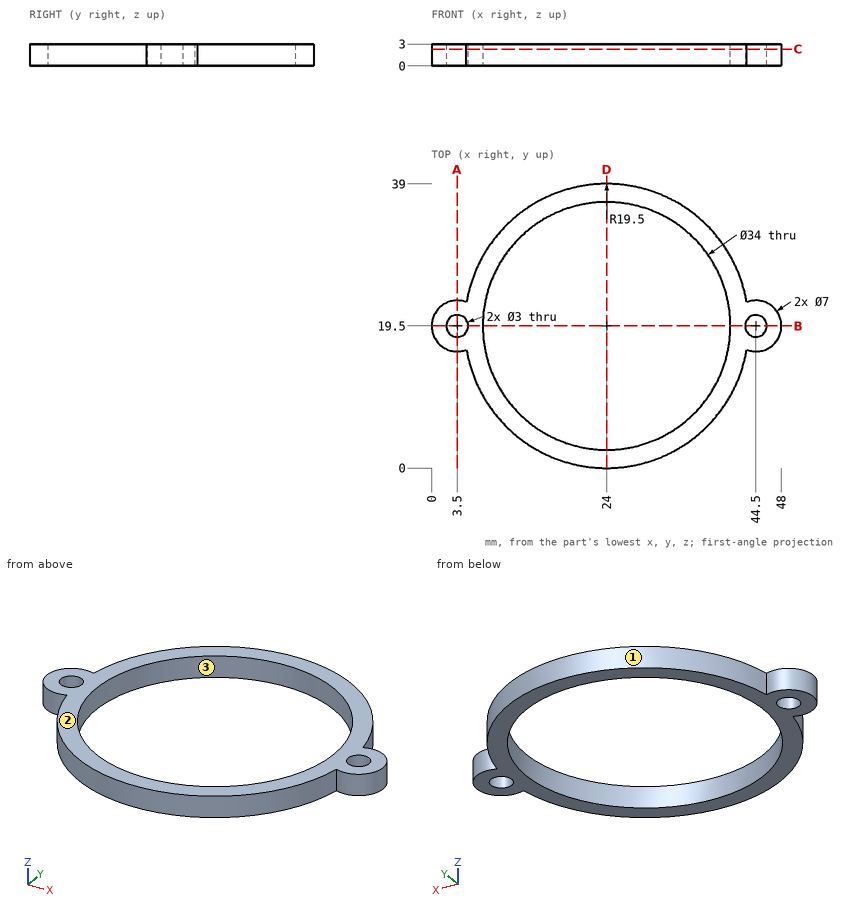
The figure shows three views and two pictorial views of one solid part (mm, origin at its lowest corner). Answer the questions. Coordinates: 2 decimals unless noted, no trailing zeros. Loops run counter-clockwise (first coordinate to the right, second up) from the corner with the lowest first, then second, coordinate; pieces in that order, holes last. Notation, with made-up numbers: (52.5, -16) -> (76.5, -16) arc R18 cw to (76.5, 19) -> close; hole circle Ø6 at (-6.5, 32.25). An arc over 180 degrees is marked (long way). Use one line per item in the form item = value. Start each with the question number.
Item 1: A flat-ended cylindrical pin translates along its axis: pin 1 Ø1 at (y, z) = (34.5, 1) entering from +X. Find the tip coordinate at first contact, or state that the pin passes through.
Item 2: The part is cut by section A-A on x = 3.5. Determine the outline of the cut face in (y, z).
Item 3: Consider L1, parallel to Y at x = 44.5, z = 0.65; L2, parallel to Y at x = 12, z = 2.45; L3, parallel to X at y = 33, z = 0.9. Determine where each line is inside the solid, lowest interval first. Write a range as [from, to].
Item 4: The part is cut by section C-C on z = 2.3. Determine the outline of the cut face in (x, y), then the cut area to 3 significant figures.
Item 5: The part is cut by section B-B on y = 19.5. Determine the outline of the cut face in (x, z).
Item 6: The mould has two halves that part along Y. Classify the marked faces 1, 2 and 3: released by +Y, released by -Y, zero draft, split by the parting line, or undercut.
Item 7: The part is cut by section D-D on x = 24. Determine the outline of the cut face in (y, z).
Answer key:
q1.pin_1 = 37.04
q2.outline = (16, 0) -> (18, 0) -> (18, 3) -> (16, 3) -> close; (21, 0) -> (23, 0) -> (23, 3) -> (21, 3) -> close
q3.L1 = [16, 18], [21, 23]
q3.L2 = [4.13, 7.46], [31.54, 34.87]
q3.L3 = [9.93, 13.67], [34.33, 38.07]
q4.outline = (4.77, 16.24) arc R19.5 ccw to (43.23, 16.24) arc R3.5 ccw (long way) to (43.23, 22.76) arc R19.5 ccw to (4.77, 22.76) arc R3.5 ccw (long way) to start; hole circle Ø3 at (3.5, 19.5); hole circle Ø34 at (24, 19.5); hole circle Ø3 at (44.5, 19.5)
q4.area = 326 mm2
q5.outline = (0, 0) -> (2, 0) -> (2, 3) -> (0, 3) -> close; (5, 0) -> (7, 0) -> (7, 3) -> (5, 3) -> close; (41, 0) -> (43, 0) -> (43, 3) -> (41, 3) -> close; (46, 0) -> (48, 0) -> (48, 3) -> (46, 3) -> close
q6.face_1 = released by +Y
q6.face_2 = zero draft
q6.face_3 = undercut
q7.outline = (0, 0) -> (2.5, 0) -> (2.5, 3) -> (0, 3) -> close; (36.5, 0) -> (39, 0) -> (39, 3) -> (36.5, 3) -> close
